Could you check a few things on this model? Use its own coordinates, in mm. Face numbers are marked on the shaded views. A direction names the side the tool comes from. Round coordinates to 2 decimals unless told otherwise and drop trailing zeros. Loops run counter-clockwise (first coordinate to the right, second up) from the corner with the lowest first, then second, coordinate; pieces in that order, holes last. Notation, with made-up numbers: (-36.75, 12.25) -> (20.25, 12.25) arc R25 ccw to (20.25, 36.25) -> close; hole circle Ø6 at (6.25, -17). An arc over 180 degrees is marked (long way). One line per item, written item: value.
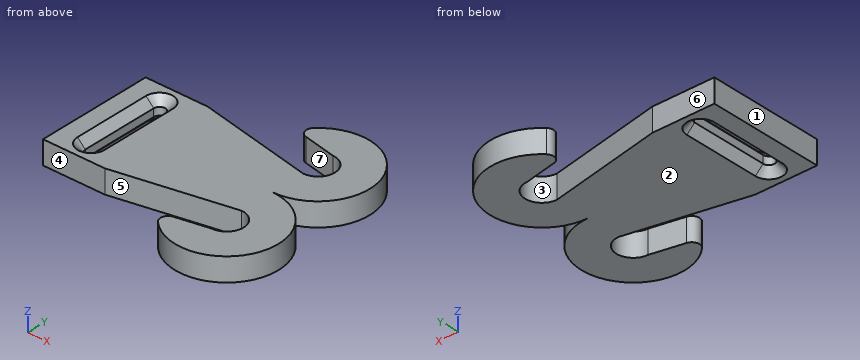
```python
from build123d import *

# Parameters (mm, degrees)
PAD_DEPTH    = 3
POCKET_DEPTH = 5
CHAMFER_SIZE = 1
FILLET_R     = 1


with BuildPart() as part:
    # Sketch → Pad (new body)
    with BuildSketch(Plane.XY):
        with BuildLine():
            Line((0, 15), (0, 0))
            Line((0, 0), (8, 0))
            Line((8, 0), (23, 3))
            ThreePointArc((23, -1.343534), (25.171767, 0.828233), (23, 3))
            Line((23, -1.343534), (17.21767, -2.5))
            ThreePointArc((17.21767, -2.5), (28.775711, -2.511474), (23, 7.5))
            ThreePointArc((23, 7.5), (28.775711, 17.511474), (17.21767, 17.5))
            Line((17.21767, 17.5), (23, 16.343534))
            ThreePointArc((23, 12), (25.171767, 14.171767), (23, 16.343534))
            Line((8, 15), (23, 12))
            Line((0, 15), (8, 15))
        make_face()
    extrude(amount=PAD_DEPTH)

    # Sketch001 (on Face13 of Pad) → Pocket (cut)
    with BuildSketch(Plane.XY.offset(3)):
        with BuildLine():
            ThreePointArc((4.75, 12.5), (4, 13.25), (3.25, 12.5))
            Line((3.25, 12.5), (3.25, 2.5))
            ThreePointArc((3.25, 2.5), (4, 1.75), (4.75, 2.5))
            Line((4.75, 12.5), (4.75, 2.5))
        make_face()
    extrude(amount=-POCKET_DEPTH, mode=Mode.SUBTRACT)

    # Chamfer
    chamfer_edges = [part.edges().sort_by_distance(p)[0] for p in [
        (3.25, 7.5, 0),
        (4.75, 7.5, 3),
    ]]
    chamfer(chamfer_edges, length=CHAMFER_SIZE)

    # Fillet
    fillet_edges = [part.edges().sort_by_distance(p)[0] for p in [
        (17.21767, -2.5, 1.5),
        (17.21767, 17.5, 1.5),
    ]]
    fillet(fillet_edges, radius=FILLET_R)


solid = part.part
```
(1) For pin 1 Ø0.9 at (x, z) = (3.5, 1.5) entering from +Y; pin 2 Ø6 at (x, y) = (19.5, 2) entering from +Z; pin 3 Ø1 at (y, z) = (17.5, 0.5) entering from -X; pin 4 Ø1.5 at (x, z) = (18.5, 1.5) entering from -Y, each with a flat end and sliding along its axis, tell me the tip position at first contact or that it passes through.
Results below:
pin 1: stops at y = 15
pin 2: stops at z = 3
pin 3: stops at x = 17.99
pin 4: stops at y = -4.69
(2) Imagine slicing it at A-A on x = 4. Write out the boundary of the cut face in (y, z).
Results below:
outline: (0, 0) -> (0.75, 0) -> (1.75, 1) -> (1.75, 2) -> (0.75, 3) -> (0, 3) -> close; (13.25, 1) -> (14.25, 0) -> (15, 0) -> (15, 3) -> (14.25, 3) -> (13.25, 2) -> close
(3) Please list where these lines run through material, in increasing order: L1, parallel to Y at x = 18.75, z = 0.6; L2, parallel to Y at x = 20.5, z = 1.05; L3, parallel to Y at x = 24, z = 1.55.
Results below:
L1: y = -4.31 to -2.19, 2.15 to 12.85, 17.19 to 19.31
L2: y = -5.36 to -1.84, 2.5 to 12.5, 16.84 to 20.36
L3: y = -5.77 to -1.1, 2.76 to 7.42, 7.58 to 12.24, 16.1 to 20.77
(4) Imagine slicing it at C-C on x = 23.75. Write out the boundary of the cut face in (y, z), then the cut area to 3 significant figures.
Results below:
outline: (-5.8, 0) -> (-1.21, 0) -> (-1.21, 3) -> (-5.8, 3) -> close; (2.87, 0) -> (7.46, 0) -> (7.46, 3) -> (2.87, 3) -> close; (7.54, 0) -> (12.13, 0) -> (12.13, 3) -> (7.54, 3) -> close; (16.21, 0) -> (20.8, 0) -> (20.8, 3) -> (16.21, 3) -> close
area: 55.1 mm²
(5) Imagine slicing it at B-B on z = 1.45. Write out the boundary of the cut face in (x, y), then the cut area to 3 significant figures.
Results below:
outline: (0, 0) -> (8, 0) -> (23, 3) arc R2.17 cw to (23, -1.34) -> (18.78, -2.19) arc R1 ccw to (18.27, -3.87) arc R6.67 ccw (long way) to (23, 7.5) arc R6.67 ccw (long way) to (18.27, 18.87) arc R1 ccw to (18.78, 17.19) -> (23, 16.34) arc R2.17 cw to (23, 12) -> (8, 15) -> (0, 15) -> close; hole (3.25, 2.5) arc R0.75 ccw to (4.75, 2.5) -> (4.75, 12.5) arc R0.75 ccw to (3.25, 12.5) -> close
area: 441 mm²
(6) Imagine slicing it at D-D on y = 5.25. Write out the boundary of the cut face in (x, z), then the cut area to 3 significant figures.
Results below:
outline: (0, 0) -> (2.25, 0) -> (3.25, 1) -> (3.25, 2) -> (2.25, 3) -> (0, 3) -> close; (4.75, 1) -> (5.75, 0) -> (28, 0) -> (28, 3) -> (5.75, 3) -> (4.75, 2) -> close
area: 77.5 mm²
(7) On a 3-axis mill with a long thin cutter (end or side, diameter ignored), from which of +Z, -Z, +X, -X, +Y, -Y can I reach the whole of each face in a straight line? I mean the marked faces 4, 5, 6 and 7. Say none if no direction works.
Results below:
face 4: +Z, -Z, -X, -Y
face 5: +Z, -Z
face 6: +Z, -Z, -X, +Y
face 7: +Z, -Z, -X
(8) We'd pull the mould along X, two halves only. Please class the marked faces 1, 2 and 3: +X half, -X half, draft (parallel to the pull), parting line (faces both ways), or undercut.
Results below:
face 1: -X half
face 2: draft
face 3: undercut
